```python
from build123d import *


with BuildPart() as f1:
    # F0 (on Front) → F1 (revolve)
    with BuildSketch(Plane.XZ):
        Polygon((-13.494493, -27.085373), (0, -27.085373), (0, 26.699817), (-3.084456, 14.940332), (-5.01224, 14.940332), (-6.940024, 16.482558), (-6.940024, 20.530906), (-9.638923, 20.530906), (-9.638923, 17.446451), (-7.51836, 12.241432), (-3.277234, 12.241432), (-3.277234, -9.735312), (-6.747246, -18.603122), (-9.446145, -18.603122), (-13.494493, -22.458691), align=None)
    revolve(axis=Axis((0, 0, -0.192778), (0, 0, -1)))


solid = f1.part
```
Geometry: final body of the model. Coordinates: model frame, mm. A direction names the side the tool comes from. Give positions to 0.01 mm unless a question says otherwise; leave off trailing zeros. Loops run counter-clockwise (first coordinate to the right, second up) from the corner with the lowest first, then second, coordinate; pieces in that order, holes last. Notation, with made-up numbers: (-11.75, -16) -> (-6.75, -16) arc R15 ccw to (-6.75, -2) -> close; hole circle Ø1 at (-0.5, 82). An arc over 180 degrees is marked (long way). Use CSV: the item, a comma, the result in double quotes.
(1) Access query for faces 1 (the face through (0.992, 7.556, 12.494)), 2 (the face through (-4.45, -8.55, 18.97)), 3 (the face through (2.925, -13.174, -24.804)). Directions: +Z, -Z, +X, -X, +Y, -Y. A direction counts if a zero-diameter tool reaches every point of the face in a straight line with its end or side. Return the directions, or none.
From the geometry:
face 1,"none"
face 2,"+Z"
face 3,"+Z, -Z"
(2) First-contact query: P1, Ø11, axis at x = 0.5, y = 0.5, coming from the +Z side; P2, Ø2, axis at y = 2.5, z = -1, coming from the +X side; P3, Ø6, axis at y = -0.5, z = -5.5, coming from the -X side; P4, Ø12, axis at x = 7.5, z = 10, coming from the -Y side. Flat tips, straight axial feed; report the tip coordinate or a pass-through.
From the geometry:
P1,"z = 26.7"
P2,"x = 2.91"
P3,"x = -3.28"
P4,"y = -7.67"
(3) Cut plane A-A (z = 18.5). Output: boundary loops of the cut face in (x, y), plus the area to 3 significant figures.
From the geometry:
outline,"circle Ø19.28 at (0, 0); circle Ø4.3 at (0, 0); hole circle Ø13.88 at (0, 0)"
area,"155 mm^2"
(4) Cut plane B-B (z = -5). Output: boundary loops of the cut face in (x, y).
From the geometry:
outline,"circle Ø6.55 at (0, 0)"
(5) Pull-direction query (Y, two-part tool) for faces 4 (the face through (-1.49, 0.47, 20.74)), 5 (the face through (2.103, -9.469, -18.844)), 6 (the face through (-3, -2, 12.241)); classes: released by +Y, released by -Y, zero draft, split by the parting line, or undercut.
From the geometry:
face 4,"undercut"
face 5,"split by the parting line"
face 6,"zero draft"
(6) Ray query, line 1 along Y through (x, z) = (0, 19.7); line 2 along Z through (x, y) = (-2.75, 6.5); line 3 along Y through (x, z) = (0, 19.25). Return the intervals inside material, ascending. Write a range as [from, to].
From the geometry:
line 1,"[-9.64, -6.94], [-1.84, 1.84], [6.94, 9.64]"
line 2,"[-27.09, -18.6], [12.24, 20.53]"
line 3,"[-9.64, -6.94], [-1.95, 1.95], [6.94, 9.64]"
